The model under review builds one solid part; all positions refer to its coordinate system, in mm. Face numbers are marked on the shaded views. A direction names the side the tool comes from. Give positions to 0.01 mm unless a question says otherwise; leave off trailing zeros. Write each loop counter-clockwise with the first axis right and the second up, starting at its lowest first coordinate (ties: lowest second). Pieces come first, ordered by that corner, then holes. Notation, with made-up numbers: M 68,-34 L 113,-34 A20 ccw 113,-25 Z; hole C 55,26.5 d1. An arc over 180 degrees is marked long. Write each question's results on one line, items separated by ' | '. Start each with the question number.
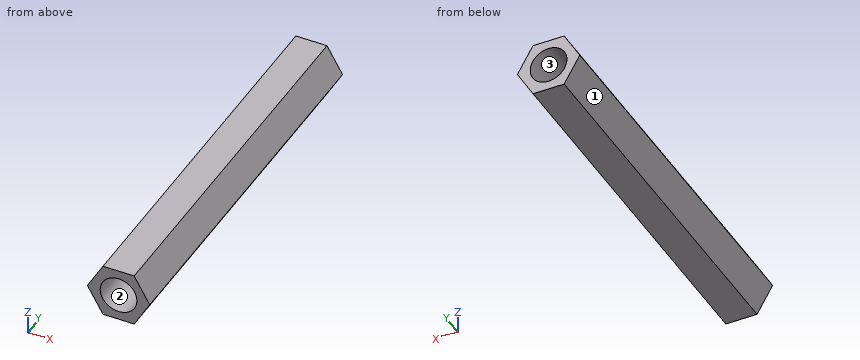
from build123d import *

# Parameters (mm, degrees)
HEX_STANDOFF_DEPTH       = 35
M3_CLEARANCE_HOLE1_D     = 3.4
M3_CLEARANCE_HOLE1_DEPTH = 5
M3_CLEARANCE_HOLE1_TIP   = 1.021463052
M3_CLEARANCE_HOLE5_D     = 3.4
M3_CLEARANCE_HOLE5_DEPTH = 5
M3_CLEARANCE_HOLE5_TIP   = 1.021463052


with BuildPart() as part:
    # Sketch1 → Hex Standoff (new body)
    with BuildSketch(Plane(origin=(0, 0, 0), x_dir=(1, 0, 0), z_dir=(0, 1, 0))):
        Polygon((-1.443375673, 2.5), (1.443375673, 2.5), (2.886751346, 0), (1.443375673, -2.5), (-1.443375673, -2.5), (-2.886751346, 0), align=None)
    extrude(amount=HEX_STANDOFF_DEPTH)

    # M3 Clearance Hole1
    with Locations(Plane(origin=(0, 35, 0), x_dir=(1, 0, 0), z_dir=(0, 1, 0))):
        with Locations((0, 0)):
            Hole(M3_CLEARANCE_HOLE1_D / 2, depth=M3_CLEARANCE_HOLE1_DEPTH)
            with Locations((0, 0, -(M3_CLEARANCE_HOLE1_DEPTH + M3_CLEARANCE_HOLE1_TIP / 2))):  # 118° drill point
                Cone(0, M3_CLEARANCE_HOLE1_D / 2, M3_CLEARANCE_HOLE1_TIP, mode=Mode.SUBTRACT)

    # M3 Clearance Hole5
    with Locations(Plane.XZ):
        with Locations((0, 0)):
            Hole(M3_CLEARANCE_HOLE5_D / 2, depth=M3_CLEARANCE_HOLE5_DEPTH)
            with Locations((0, 0, -(M3_CLEARANCE_HOLE5_DEPTH + M3_CLEARANCE_HOLE5_TIP / 2))):  # 118° drill point
                Cone(0, M3_CLEARANCE_HOLE5_D / 2, M3_CLEARANCE_HOLE5_TIP, mode=Mode.SUBTRACT)


solid = part.part
(1) Wall thickness on L1, parallel to Z at x = -0.9, y = 2.5; L2, parallel to Z at x = 0, y = 32.6; L3, parallel to X at y = 31.5, z = 0.45: over which ranges is each line inside the solid? List them lowest first.
(2) Add section B-B (y = 24.5). State the section outline as (x, z) points, then the cut area to 3 significant figures.
(3) Add section A-A (y = 32). State the section outline as (x, z) points.
(4) Add section C-C (x = 2.1). State the section outline as (y, z) points.
(5) Add section D-D (x = -2.15). State the section outline as (y, z) points, then the cut area to 3 significant figures.
(6) Clearance check with flat-ended pins moving along their axes: P1, Ø2, axis at x = 0, z = 0, coming from the -Y side; P2, Ø2.5, axis at x = 0, z = 0, coming from the +Y side; P3, Ø2, axis at y = 26, z = -1.5, coming from the +X side. State where each tip first meets the part, or that it passes through.
(7) Machinability: for the marked faces 1, 2 and 3, which of the approach directions +Z, -Z, +X, -X, +Y, -Y give a long, thin tool a straight path to every point of the face, cutting with its end or side? Answer none if there is none.
Calculated:
1) L1: z = -2.5 to -1.44, 1.44 to 2.5 | L2: z = -2.5 to -1.7, 1.7 to 2.5 | L3: x = -2.63 to -1.64, 1.64 to 2.63
2) outline: M -2.89,0 L -1.44,-2.5 L 1.44,-2.5 L 2.89,0 L 1.44,2.5 L -1.44,2.5 Z | area: 21.7 mm²
3) outline: M -2.89,0 L -1.44,-2.5 L 1.44,-2.5 L 2.89,0 L 1.44,2.5 L -1.44,2.5 Z; hole C 0,0 d3.4
4) outline: M 0,-1.36 L 35,-1.36 L 35,1.36 L 0,1.36 Z
5) outline: M 0,-1.28 L 35,-1.28 L 35,1.28 L 0,1.28 Z | area: 89.3 mm²
6) P1: stops at y = 5.42 | P2: stops at y = 29.73 | P3: stops at x = 2.6
7) face 1: -Z, -X, +Y, -Y | face 2: -Y | face 3: +Y
